from build123d import *

# Parameters (mm, degrees)
SKETCH1_R           = 82
BOSS_EXTRUDE1_DEPTH = 8
SKETCH2_R           = 2
CUT_EXTRUDE1_DEPTH  = 8
CIRPATTERN1_COUNT   = 4
SKETCH3_R           = 4
SKETCH3_R_2         = 1.25
CUT_EXTRUDE2_DEPTH  = 10
CUT_EXTRUDE3_DEPTH  = 3.2
SKETCH5_R           = 1
CUT_EXTRUDE4_DEPTH  = 12
CIRPATTERN2_COUNT   = 4
CIRPATTERN3_COUNT   = 4


with BuildPart() as part:
    # Sketch1 → Boss-Extrude1 (new body)
    with BuildSketch(Plane.XY):
        Circle(SKETCH1_R)
    extrude(amount=BOSS_EXTRUDE1_DEPTH)

    # Sketch2 → Cut-Extrude1 (cut)
    with BuildSketch(Plane.XY.offset(8)):
        with Locations((0, 60)):
            Circle(SKETCH2_R)
    cut_extrude1 = extrude(amount=-CUT_EXTRUDE1_DEPTH, mode=Mode.SUBTRACT)

    # CirPattern1: Cut-Extrude1 ×4 about axis
    cirpattern1_axis = Axis((0, 0, 0), (0, 0, 1))
    for i in range(1, CIRPATTERN1_COUNT):
        add(cut_extrude1.rotate(cirpattern1_axis, i * 360 / CIRPATTERN1_COUNT), mode=Mode.SUBTRACT)

    # Sketch3 → Cut-Extrude2 (cut)
    with BuildSketch(Plane.XY.offset(8)):
        Circle(SKETCH3_R)
        with Locations((0, 8.38)):
            Circle(SKETCH3_R_2)
        with Locations((0, -19.13)):
            Circle(SKETCH3_R_2)
    extrude(amount=-CUT_EXTRUDE2_DEPTH, mode=Mode.SUBTRACT)

    # Sketch4 → Cut-Extrude3 (cut)
    with BuildSketch(Plane(origin=(0, 0, 0), x_dir=(-1, 0, 0), z_dir=(0, 0, -1))):
        Polygon((-162.322467781, -20.961900653), (-166.013325515, -22.608382515), (-166.432859263, -26.628000005), (-163.161535277, -29.001135634), (-159.470677543, -27.354653772), (-159.051143795, -23.335036282), align=None)
        Polygon((-64.01961749, 0.419533748), (-62.373135629, -3.271323986), (-58.353518138, -3.690857734), (-55.98038251, -0.419533748), (-57.626864371, 3.271323986), (-61.646481862, 3.690857734), align=None)
        Polygon((-183.703902182, 77.340949637), (-185.350384043, 81.031807371), (-189.370001534, 81.451341119), (-191.743137162, 78.180017133), (-190.0966553, 74.489159399), (-186.07703781, 74.069625651), align=None)
        Polygon((-85.401051891, 98.722384038), (-81.710194157, 100.3688659), (-81.290660409, 104.38848339), (-84.561984395, 106.761619019), (-88.252842129, 105.115137157), (-88.672375877, 101.095519667), align=None)
    cut_extrude3 = extrude(amount=-CUT_EXTRUDE3_DEPTH, mode=Mode.SUBTRACT)

    # Sketch5 → Cut-Extrude4 (cut)
    with BuildSketch(Plane(origin=(-57.982756057, 57.982756057, 0), x_dir=(0.7071067811865477, 0.7071067811865475, 0), z_dir=(-0.7071067811865475, 0.7071067811865477, 0))):
        with Locations(Location((0, -4, 0), (0, 0, 180))):
            Circle(SKETCH5_R)
    cut_extrude4 = extrude(amount=-CUT_EXTRUDE4_DEPTH, mode=Mode.SUBTRACT)

    # CirPattern2: Cut-Extrude4 ×4 about axis
    cirpattern2_axis = Axis((0, 0, 0), (0, 0, 1))
    for i in range(1, CIRPATTERN2_COUNT):
        add(cut_extrude4.rotate(cirpattern2_axis, i * 360 / CIRPATTERN2_COUNT), mode=Mode.SUBTRACT)

    # CirPattern3: Cut-Extrude3 ×4 about axis
    cirpattern3_axis = Axis((0, 0, 0), (0, 0, 1))
    for i in range(1, CIRPATTERN3_COUNT):
        add(cut_extrude3.rotate(cirpattern3_axis, i * 360 / CIRPATTERN3_COUNT), mode=Mode.SUBTRACT)


solid = part.part
Could you check a few things on this model? Use its own coordinates, in mm. A direction names the side the tool comes from. Give positions to 0.01 mm unless a question says otherwise; leave off trailing zeros. Order: outer loops, then holes, each group sorted by start corner. A loop starts at its lowest first (then second) coordinate and runs counter-clockwise, first axis right, second up.
1. Suppose I cut it at B-B (x = -20). List the corners of the cut face in (y, z) for me.
2. We'd pull the mould along Z, two halves only. Please class faces 3 (the cylindrical face through (-54.32, -53.28, 4.68)), 4 (the cylindrical face through (0, -62, 6)), 5 (the flat face through (17, 1, 0)): pulls with the +Z half, pulls with the -Z half, needs draft (parallel to the pull), parting line crosses it, or undercut.
3. For faces 1 (the cylindrical face through (-0.867, -3.905, 4.056)), 2 (the flat face through (1, -62, 3.2)), which set-ups out of +Z, -Z, +X, -X, +Y, -Y let a thin tool reach every point of the face, with its end or its side?
4. Will these pins go through, and if not, where does the flat tip stop? P1, Ø2, axis at y = 65, z = 1.5, coming from the +X side; P2, Ø2.5, axis at x = 60, y = 0, coming from the +Z side; P3, Ø3, axis at x = -12, z = 1.5, coming from the +Y side; P4, Ø2, axis at x = -1, y = 62, coming from the -Z side.
5. Suppose I cut it at C-C (y = 68.5). List the corners of the cut face in (x, z) for me, plus the area to 3 significant figures.
6. Suppose I cut it at A-A (z = 1.25). List the corners of the cut face in (x, y) for me.
7. I need wall thicknesses on L1, parallel to Y at x = 0, z = 4.55; L2, parallel to Z at x = -57.5, y = -56.5; L3, parallel to Y at x = -60, z = 2. Which ranges of each line are inside material? Lowest first, please.
Solved:
1. outline: (-79.52, 0) - (79.52, 0) - (79.52, 8) - (-79.52, 8) - close
2. face 3: undercut
2. face 4: needs draft
2. face 5: pulls with the -Z half
3. face 1: +Z, -Z
3. face 2: -Z
4. P1: stops at x = 51.26
4. P2: passes through
4. P3: stops at y = 81.32
4. P4: stops at z = 3.2
5. outline: (-45.07, 0) - (45.07, 0) - (45.07, 8) - (-45.07, 8) - close
5. area: 721 mm2
6. outline: circle Ø164 at (0, 0); hole (-64.02, -0.42) - (-61.65, -3.69) - (-57.63, -3.27) - (-55.98, 0.42) - (-58.35, 3.69) - (-62.37, 3.27) - close; hole circle Ø8 at (0, 0); hole (-3.69, -58.35) - (-3.27, -62.37) - (0.42, -64.02) - (3.69, -61.65) - (3.27, -57.63) - (-0.42, -55.98) - close; hole (-3.69, 61.65) - (-3.27, 57.63) - (0.42, 55.98) - (3.69, 58.35) - (3.27, 62.37) - (-0.42, 64.02) - close; hole circle Ø2.5 at (0, -19.13); hole circle Ø2.5 at (0, 8.38); hole (55.98, -0.42) - (58.35, -3.69) - (62.37, -3.27) - (64.02, 0.42) - (61.65, 3.69) - (57.63, 3.27) - close
7. L1: y = -82 to -62, -58 to -20.38, -17.88 to -4, 4 to 7.13, 9.63 to 58, 62 to 82
7. L2: z = 0 to 3.29, 4.71 to 8
7. L3: y = -55.89 to -3.52, 3.52 to 55.89
